Part model, mm, in its own coordinate system. Give positions to 0.01 mm unless a question says otherwise; leave off trailing zeros. Order: outer loops, then holes, each group sorted by start corner. A loop starts at its lowest first (then second) coordinate and runs counter-clockwise, first axis right, second up.
1. Slice it at C-C on z = 4. List the corners of the cut face in (x, y).
2. Mould opens along Z. For faces 1 (the cylindrical face through (31.661, 0.016, 5.831)), 2 (the flat face through (32, -4.875, 1)), 3 (the flat face through (32, 1, -8.46)), 4 (the cylindrical face through (29.855, 1.387, -0.902)) say: +Z half, -Z half, draft (parallel to the pull), parting line (faces both ways), or undercut.
3. Probe line 1 (Z direction, x = 31.75, y = -1.5); line 2 (Z direction, x = 32.25, y = 0); line 3 (Z direction, x = 31.75, y = 3). List the from-to ranges inside material, lowest first.
4. Slice it at A-A on y = 2. List the corners of the cut face in (x, z).
5. Slice it at D-D on y = -2. List the corners of the cut face in (x, z), and give its area (3 significant figures).
6. Drop a flat-ended pin along its axis: pin 1 Ø6 at (x, z) = (31.75, -2.11) entering from +Y. Give the stop position or say it passes through.
7. Slice it at B-B on x = 33.5. List the corners of the cut face in (y, z), and give its area (3 significant figures).
Autodesk Inventor part; units mm, degrees
ref_plane "YZ Plane" through (0, 0, 0) normal (1, 0, 0) x (0, 1, 0)
ref_plane "XZ Plane" through (0, 0, 0) normal (0, 1, 0) x (-1, 0, 0)
ref_plane "XY Plane" through (0, 0, 0) normal (0, 0, 1) x (1, 0, 0)
sketch "Sketch1" plane through (0, 0, 0) normal (1, 0, 0) x (0, 1, 0)
  line L0 (7.8254, 10.5896) -> (-4.8746, 10.5896)
  line L1 (-4.8746, 10.5896) -> (-4.8746, -8.4604)
  line L2 (-4.8746, -8.4604) -> (7.8254, -8.4604)
  line L3 (7.8254, -8.4604) -> (7.8254, 10.5896)
  point P0 (0, 0)
  dimension "d0" = 19.05
  dimension "d1" = 12.7
extrude "Extrusion1" add sketch "Sketch1" along normal blind 38.1
sketch "Sketch2" plane through (38.1, 0, 0) normal (1, 0, 0) x (0, 0, -1)
  line L0 (-10.5896, 7.8254) -> (-10.5896, -4.8746)
  line L1 (8.4604, 7.8254) -> (-10.5896, 7.8254)
  point P0 (0, 0)
  point P1 (-4.2396, 1.4754)
  dimension "d4" = 6.35
  dimension "d5" = 6.35
hole "Hole1" at (38.1, 1.4754, 4.2396) direction (-1, 0, 0) diameter 4.318 end through all
sketch "Sketch3" plane through (0, 7.8254, 10.5896) normal (0, 1, 0) x (1, 0, 0)
  line L0 (38.1, 19.05) -> (38.1, 0)
  line L1 (0, 19.05) -> (0, 0)
  line L2 (0, 19.05) -> (38.1, 19.05)
  point P0 (0, 10.5896)
  point P1 (6.35, 12.7)
  point P2 (31.75, 12.7)
  dimension "d13" = 6.35
  dimension "d14" = 6.35
  dimension "d15" = 6.35
  dimension "d16" = 0
hole "Hole2" at (6.35, 7.8254, -2.1104) at (31.75, 7.8254, -2.1104) direction (0, -1, 0) diameter 4.4958 end through all
sketch "Sketch4" plane through (0, 7.8254, 10.5896) normal (0, 1, 0) x (1, 0, 0)
  line L0 (-8.5328, 26.8788) -> (25.4, 26.8788)
  line L1 (25.4, 26.8788) -> (25.4, -5.2507)
  line L2 (25.4, -5.2507) -> (-8.5328, -5.2507)
  line L3 (-8.5328, -5.2507) -> (-8.5328, 26.8788)
  line L4 (0, 19.05) -> (0, 0)
  point P0 (0, 10.5896)
  dimension "d24" = 25.4
extrude "Extrusion2" cut sketch "Sketch4" against normal blind 112.7125
properties part number "MotorSpacerBlock3"
Data:
1. outline: (25.4, -4.87) - (38.1, -4.87) - (38.1, -0.67) - (25.4, -0.67) - close; (25.4, 3.62) - (38.1, 3.62) - (38.1, 7.83) - (25.4, 7.83) - close
2. face 1: undercut
2. face 2: draft
2. face 3: -Z half
2. face 4: undercut
3. line 1: z = -8.46 to -4.36, 0.14 to 10.59
3. line 2: z = -8.46 to -4.3, 0.08 to 2.66, 5.82 to 10.59
3. line 3: z = -8.46 to -4.36, 0.14 to 2.71, 5.77 to 10.59
4. outline: (25.4, -8.46) - (38.1, -8.46) - (38.1, 2.15) - (25.4, 2.15) - close; (25.4, 6.33) - (38.1, 6.33) - (38.1, 10.59) - (25.4, 10.59) - close; hole circle Ø4.5 at (31.75, -2.11)
5. outline: (25.4, -8.46) - (38.1, -8.46) - (38.1, 10.59) - (25.4, 10.59) - close; hole circle Ø4.5 at (31.75, -2.11)
5. area: 226 mm2
6. pin 1: stops at y = 7.83
7. outline: (-4.87, -8.46) - (7.83, -8.46) - (7.83, -3.52) - (-4.87, -3.52) - close; (-4.87, -0.7) - (7.83, -0.7) - (7.83, 10.59) - (-4.87, 10.59) - close; hole circle Ø4.32 at (1.48, 4.24)
7. area: 191 mm2
